Design review of the part shown in the three views and the two pictorial views. Dimensions are in mm from the part's minimum x, y and z. Coordinates: 2 decimals unless noted, no trailing zeros. Loops run counter-clockwise (first coordinate to the right, second up) from the corner with the lowest first, then second, coordinate; pieces in that order, holes last.
Q1. Wall thickness on probe 1 along Z at (x, y) = (14.5, 4.85); probe 2 along Z at (x, y) = (14.5, 2.6); probe 3 along Z at (x, y) = (9, 5.5): over which ranges is each line inside the solid? List them lowest first.
Q2. Draft analysis for pull direction Y (two halves, no side actions). For the marked faces 1, 2 and 3, state which applies: released by +Y, released by -Y, zero draft, split by the parting line, or undercut.
Q3. For P1, Ø2, axis at x = 4, y = 2.5, coming from the +Z side; P2, Ø1.5, axis at y = 4.5, z = 13, coming from the -X side; P3, Ø2, axis at x = 12.5, y = 1.5, coming from the -Z side, all flat-tipped, find the tip position at first contact; note any pin that passes through.
Q4. Add section A-A on z = 14.5. Give the boundary of the cut face in (x, y), and give its area (4 significant figures).
Q5. Add section C-C on z = 4.5. Give the boundary of the cut face in (x, y).
Q6. Add section D-D on y = 3. Give the boundary of the cut face in (x, z), and give its area (3 significant figures).
Q7. Add section B-B on x = 14.5. Give the boundary of the cut face in (y, z), and give its area (4 significant figures).
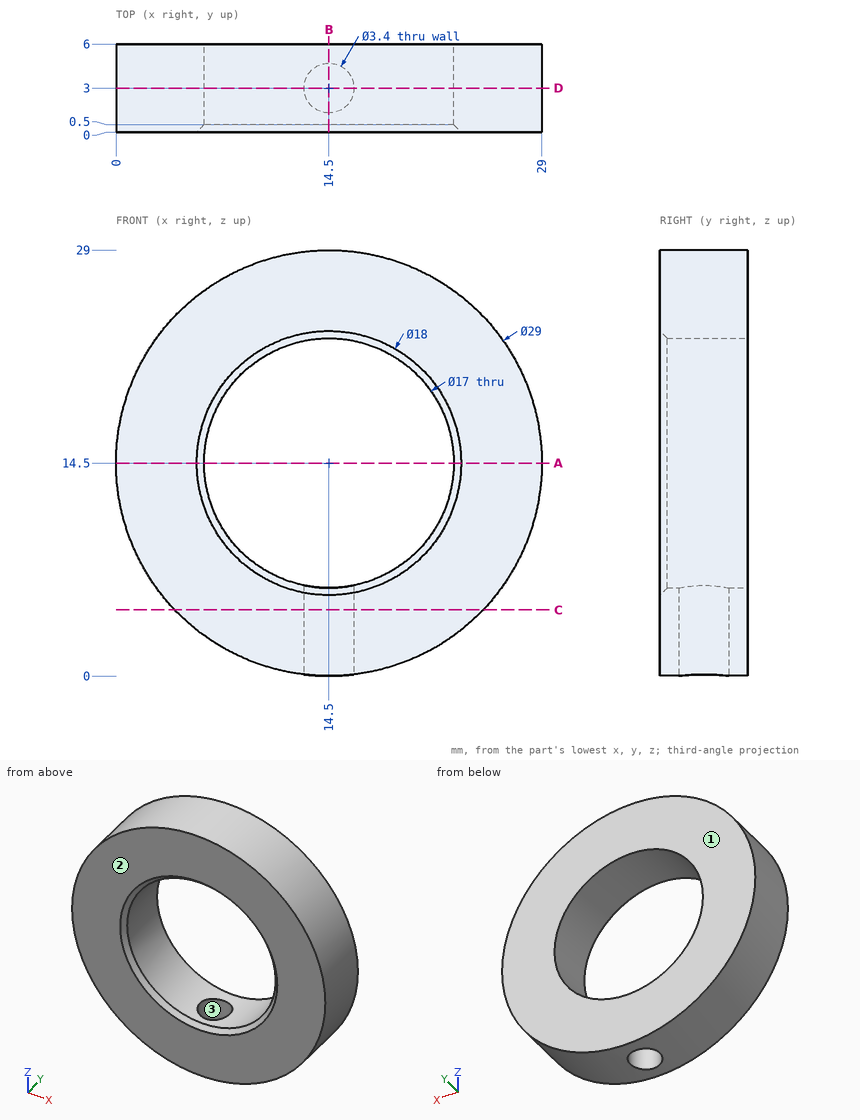
Entries:
1. probe 1: z = 0 to 6, 23 to 29
1. probe 2: z = 23 to 29
1. probe 3: z = 1.08 to 8.02, 20.98 to 27.92
2. face 1: released by +Y
2. face 2: released by -Y
2. face 3: undercut
3. P1: stops at z = 25.45
3. P2: stops at x = 0.02
3. P3: stops at z = 0.03
4. outline: (0, 0) - (5.5, 0) - (6, 0.5) - (6, 6) - (0, 6) - close; (23, 0.5) - (23.5, 0) - (29, 0) - (29, 6) - (23, 6) - close
4. area: 71.75 mm2
5. outline: (4, 0) - (25, 0) - (25, 6) - (4, 6) - close; hole circle Ø3.4 at (14.5, 3)
6. outline: (12.8, 0.1) - (12.8, 6.17) arc R8.5 cw (long way) to (16.2, 6.17) - (16.2, 0.1) arc R14.5 ccw (long way) to start
6. area: 413 mm2
7. outline: (0, 0) - (1.3, 0) - (1.3, 6) - (0.5, 6) - (0, 5.5) - close; (0, 23.5) - (0.5, 23) - (6, 23) - (6, 29) - (0, 29) - close; (4.7, 0) - (6, 0) - (6, 6) - (4.7, 6) - close
7. area: 51.35 mm2
